from build123d import *

# Parameters (mm, degrees)
EXTRUDE_1_DEPTH     = 1
EXTRUDE_2_DEPTH     = 6
SKETCH_3_R          = 2
CUT_EXTRUDE_1_DEPTH = 1
EXTRUDE_3_DEPTH     = 2
EXTRUDE_4_DEPTH     = 1
SKETCH_6_R          = 1.5
CUT_EXTRUDE_2_DEPTH = 1


with BuildPart() as part:
    # 草图1 → 凸台-拉伸1 (new body)
    with BuildSketch(Plane(origin=(0, 0, 0), x_dir=(1, 0, 0), z_dir=(0, 1, 0))):
        Polygon((23.47582205, -4.484524381), (23.47582205, -14.484524381), (16.47582205, -14.484524381), (16.47582205, -15.484524381), (2.97582205, -15.484524381), (2.97582205, -22.484524381), (-4.02417795, -22.484524381), (-4.02417795, -15.484524381), (-14.52417795, -15.484524381), (-14.52417795, -3.484524381), (-4.02417795, -3.484524381), (-4.02417795, 3.515475619), (2.97582205, 3.515475619), (2.97582205, -3.484524381), (16.47582205, -3.484524381), (16.47582205, -4.484524381), align=None)
        Polygon((-12.52417795, -6.484524381), (-12.52417795, -12.484524381), (-6.02417795, -12.484524381), (-5.02417795, -11.484524381), (-5.02417795, -6.484524381), align=None, mode=Mode.SUBTRACT)
    extrude(amount=EXTRUDE_1_DEPTH)

    # 草图2 → 凸台-拉伸2 (add)
    with BuildSketch(Plane.XZ):
        Polygon((-13.52417795, 5.484524381), (-13.52417795, 13.484524381), (-5.609964387, 13.484524381), (-4.02417795, 11.898737944), (-4.02417795, 5.484524381), align=None)
        Polygon((-12.52417795, 12.484524381), (-6.02417795, 12.484524381), (-5.02417795, 11.484524381), (-5.02417795, 6.484524381), (-12.52417795, 6.484524381), align=None, mode=Mode.SUBTRACT)
    extrude(amount=EXTRUDE_2_DEPTH)

    # 草图3 → 切除-拉伸1 (cut)
    with BuildSketch(Plane(origin=(0, 1, 0), x_dir=(1, 0, 0), z_dir=(0, 1, 0))):
        with Locations(Location((-0.24417795, -9.484524381, 0), (0, 0, 270))):
            Circle(SKETCH_3_R)
    extrude(amount=-CUT_EXTRUDE_1_DEPTH, mode=Mode.SUBTRACT)

    # 草图4 → 凸台-拉伸3 (add)
    with BuildSketch(Plane(origin=(0, 1, 0), x_dir=(1, 0, 0), z_dir=(0, 1, 0))):
        Polygon((-14.52417795, -3.484524381), (16.47582205, -3.484524381), (16.47582205, -4.484524381), (-13.52417795, -4.484524381), (-13.52417795, -14.484524381), (16.47582205, -14.484524381), (16.47582205, -15.484524381), (-14.52417795, -15.484524381), align=None)
    extrude(amount=EXTRUDE_3_DEPTH)

    # 草图5 → 凸台-拉伸4 (add)
    with BuildSketch(Plane(origin=(0, 3, 0), x_dir=(1, 0, 0), z_dir=(0, 1, 0))):
        Polygon((-14.52417795, -3.484524381), (-14.52417795, -15.484524381), (-4.02417795, -15.484524381), (-4.02417795, -12.804524381), (-6.72417795, -12.804524381), (-6.72417795, -10.304524381), (-4.02417795, -10.304524381), (-4.02417795, -3.484524381), align=None)
    extrude(amount=EXTRUDE_4_DEPTH)

    # 草图6 → 切除-拉伸2 (cut)
    with BuildSketch(Plane(origin=(0, 1, 0), x_dir=(1, 0, 0), z_dir=(0, 1, 0))):
        with Locations(Location((-0.52417795, 0.515475619, 0), (0, 0, 270))):
            Circle(SKETCH_6_R)
        with Locations(Location((-0.52417795, -19.484524381, 0), (0, 0, 90))):
            Circle(SKETCH_6_R)
    extrude(amount=-CUT_EXTRUDE_2_DEPTH, mode=Mode.SUBTRACT)


solid = part.part
The model under review builds one solid part; all positions refer to its coordinate system, in mm. A direction names the side the tool comes from. Coordinates: 2 decimals unless noted, no trailing zeros. Loops run counter-clockwise (first coordinate to the right, second up) from the corner with the lowest first, then second, coordinate; pieces in that order, holes last. Notation, with made-up numbers: (59.5, -17.75) -> (105.5, -17.75) arc R33 ccw to (105.5, 21.25) -> close; hole circle Ø6 at (-3.75, 69.25). An arc over 180 degrees is marked (long way). Use a Markdown table: item, result. Add a question column.
1. To check wall thickness, follow line 1 (X direction, y = -5, z = 11); line 2 (Z direction, x = -2.5, y = 2.25); line 3 (X direction, y = 2.25, z = 5.5). State the ranges of each line that lie inside material, in increasing order.
2. Add section B-B on x = 11. Write out the cut boundary in (y, z).
3. Draft analysis for pull direction Z (two halves, no side actions). For faces 1 (the face through (19.9, 0.5, 4.485)), 2 (the face through (-13.524, 2, 9)), 3 (the face through (-5.53, -2.45, 11.99)), 4 (the face through (-0.5, 0.5, 22.485)), state which applies: pulls with the +Z half, pulls with the -Z half, needs draft (parallel to the pull), parting line crosses it, or undercut.
4. Machinability: for faces 5 (the face through (-4.024, 0.5, 19)), 6 (the face through (-12.524, -2, 9)), 7 (the face through (-10, -3, 13.485)), 8 (the face through (-4.024, 3.5, 14.2)), which of the approach directions +Z, -Z, +X, -X, +Y, -Y give a long, thin tool a straight path to every point of the face, cutting with its end or side? Answer none if there is none.
5. Add section A-A on y = 3.5. Write out the cut boundary in (x, z).
6. Add section D-D on y = -3.5. Write out the cut boundary in (x, z).
7. Clearance check with flat-ended pins moving along their axes: pin 1 Ø0.5 at (y, z) = (2, 15) entering from +X; pin 2 Ø3 at (y, z) = (-4.5, 13) entering from +X; pin 3 Ø1.5 at (x, z) = (-7.5, 8.5) entering from -Y. State where each tip first meets the part, or that it passes through.
8. Add section C-C on z = 6. Write out the cut boundary in (x, y), plus the area to 4 significant figures.
Returned:
| question | item | result |
|---|---|---|
| 1 | line 1 | x = -13.52 to -12.52, -5.02 to -4.02 |
| 1 | line 2 | z = 3.48 to 4.48, 14.48 to 15.48 |
| 1 | line 3 | x = -14.52 to -13.52 |
| 2 | outline | (0, 3.48) -> (3, 3.48) -> (3, 4.48) -> (1, 4.48) -> (1, 14.48) -> (3, 14.48) -> (3, 15.48) -> (0, 15.48) -> close |
| 3 | face 1 | pulls with the -Z half |
| 3 | face 2 | undercut |
| 3 | face 3 | undercut |
| 3 | face 4 | pulls with the +Z half |
| 4 | face 5 | +Z, -X, +Y, -Y |
| 4 | face 6 | -Y |
| 4 | face 7 | +Z, +X, -X, -Y |
| 4 | face 8 | +Z, -Z, +X, +Y |
| 5 | outline | (-14.52, 3.48) -> (-4.02, 3.48) -> (-4.02, 10.3) -> (-6.72, 10.3) -> (-6.72, 12.8) -> (-4.02, 12.8) -> (-4.02, 15.48) -> (-14.52, 15.48) -> close |
| 6 | outline | (-13.52, 5.48) -> (-4.02, 5.48) -> (-4.02, 11.9) -> (-5.61, 13.48) -> (-13.52, 13.48) -> close; hole (-12.52, 6.48) -> (-5.02, 6.48) -> (-5.02, 11.48) -> (-6.02, 12.48) -> (-12.52, 12.48) -> close |
| 7 | pin 1 | stops at x = 16.48 |
| 7 | pin 2 | stops at x = -4.02 |
| 7 | pin 3 | stops at y = 3 |
| 8 | outline | (-14.52, 0) -> (-13.52, 0) -> (-13.52, -6) -> (-4.02, -6) -> (-4.02, 0) -> (23.48, 0) -> (23.48, 1) -> (-13.52, 1) -> (-13.52, 3) -> (-4.02, 3) -> (-4.02, 4) -> (-14.52, 4) -> close |
| 8 | area | 107.5 mm² |
